Check sheet for the modelled part. Datum: model origin and axes. Units: mm. A direction names the side the tool comes from. Give positions to 0.01 mm unless a question says otherwise; leave off trailing zeros. Loops run counter-clockwise (first coordinate to the right, second up) from the corner with the lowest first, then second, coordinate; pieces in that order, holes last. Notation, with made-up numbers: (30.25, 55.25) - (69.25, 55.25) arc R11 ccw to (69.25, 72.25) - close; hole circle Ø2 at (77, 7). An arc over 180 degrees is marked (long way). Answer in a Markdown table with one row per item. Add a question column.
(1) Sectioned sample at C-C on x = -12. Enter the section's corners in (y, z).
(2) Sectioned sample at A-A on y = 10. Enter the section's corners in (x, z), then the cut area to 3 significant figures.
(3) Thickness scan on L1, parallel to X at y = -52, z = 69; L2, parallel to Y at x = -12, z = -12; L3, parallel to Y at x = -41.5, z = 22.5. Record the ranges inside material, lowest first.
(4) Sectioned sample at D-D on z = -18. Enter the section's corners in (x, y), then the cut area to 3 significant figures.
(5) Sectioned sample at B-B on z = 73. Enter the section's corners in (x, y).
(6) Set-up check for faces 4 (the face through (-38, 66.514, 29)), 5 (the face through (-13, -13, -8.321)), 6 (the face through (0, 16, 18)): record each of +Z, -Z, +X, -X, +Y, -Y from which the full face is reachable in a straight line by a thin tool's end or side.
(7) Go/stop test with flat-tipped pins: P1, Ø12.5, axis at x = 15, z = 24.5, coming from the -Y side; P2, Ø2, axis at x = 3, y = -27, coming from the +Z side; P3, Ø12.5, axis at x = -7, z = -55.5, coming from the +Y side. Record where each tip stops, or that it passes through.
(8) Draft check along Z on faces 1 (the face through (-25.4, -7, 46)), 2 (the face through (0, -13, -14)), 3 (the face through (-38, -9, 102.951)). Enter one of: released by +Z, released by -Z, zero draft, split by the parting line, or undercut.
from build123d import *

# Parameters (mm, degrees)
F0_W     = 75.5894184113
F0_H     = 75.1656368375
F0_W_2   = 75.6931006908
F1_DEPTH = 25.4
F2_W     = 58.5926715285
F2_H     = 41.5871664882
F2_W_2   = 8.5760951042
F2_H_2   = 8.3214826882
F2_W_3   = 8.4206517786
F3_DEPTH = 25.4
F4_W     = 91.1564920098
F4_H     = 141.0772651434
F4_H_2   = 8.5697695613
F5_DEPTH = 25.4


with BuildPart() as f1:
    # F0 (on Right) → F1 (new body)
    with BuildSketch(Plane.YZ):
        with Locations((-37.7947092056, 37.5828184187)):
            Rectangle(F0_W, F0_H)
        with Locations((37.8465503454, 37.5828184187)):
            Rectangle(F0_W_2, F0_H)
        Polygon((0, 0), (-75.5894184113, 0), (-75.5894184113, -74.7117847204), (75.6931006908, -74.7117847204), (75.6931006908, 0), align=None)
    extrude(amount=F1_DEPTH)

    # F2 (on face) → F3 (join)
    with BuildSketch(Plane(origin=(0, 0, 0), x_dir=(0, -1, 0), z_dir=(-1, 0, 0))):
        with Locations((46.293082647, -53.9182014763)):
            Rectangle(F2_W, F2_H)
        Polygon((0, -74.7117847204), (16.9967468828, -74.7117847204), (16.9967468828, -33.1246182323), (16.9967468828, -22.4458947778), (0, -22.4458947778), align=None)
        Polygon((16.9967468828, -33.1246182323), (75.5894184113, -33.1246182323), (75.5894184113, -20.1201699674), (16.9967468828, -20.1201699674), (16.9967468828, -22.4458947778), align=None)
        Polygon((16.9967468828, -20.1201699674), (75.5894184113, -20.1201699674), (75.5894184113, 0), (16.9967468828, 0), (16.9967468828, -8.3214826882), align=None)
        Polygon((0, -22.4458947778), (16.9967468828, -22.4458947778), (16.9967468828, -20.1201699674), (8.5760951042, -20.1201699674), (8.5760951042, -8.3214826882), (0, -8.3214826882), align=None)
        with Locations((4.2880475521, -4.1607413441)):
            Rectangle(F2_W_2, F2_H_2)
        with Locations((12.7864209935, -4.1607413441)):
            Rectangle(F2_W_3, F2_H_2)
    extrude(amount=F3_DEPTH)

    # F4 (on face) → F5 (join)
    with BuildSketch(Plane(origin=(-25.4, 0, 0), x_dir=(0, -1, 0), z_dir=(-1, 0, 0))):
        with Locations((-20.9354860708, 23.8422006369)):
            Rectangle(F4_W, F4_H)
        Polygon((24.6427599341, 102.9506027699), (24.6427599341, 94.3808332086), (24.6427599341, -46.6964319348), (82.840628922, -46.6964319348), (82.840628922, 102.9506027699), align=None)
        with Locations((-20.9354860708, 98.6657179892)):
            Rectangle(F4_W, F4_H_2)
    extrude(amount=F5_DEPTH)


solid = f1.part
Reply:
| question | item | result |
|---|---|---|
| 1 | outline | (-75.59, -74.71) - (0, -74.71) - (0, 0) - (-75.59, 0) - close; hole (-17, -20.12) - (-8.58, -20.12) - (-8.58, -8.32) - (-17, -8.32) - close |
| 2 | outline | (-50.8, -46.7) - (-25.4, -46.7) - (-25.4, 102.95) - (-50.8, 102.95) - close; (0, -74.71) - (25.4, -74.71) - (25.4, 75.17) - (0, 75.17) - close |
| 2 | area | 7,610 mm^2 |
| 3 | L1 | -50.8 to -25.4, 0 to 25.4 |
| 3 | L2 | -75.59 to -17, -8.58 to 0 |
| 3 | L3 | -82.84 to 66.51 |
| 4 | outline | (-50.8, -82.84) - (-25.4, -82.84) - (-25.4, -75.59) - (25.4, -75.59) - (25.4, 75.69) - (0, 75.69) - (0, 0) - (-25.4, 0) - (-25.4, 66.51) - (-50.8, 66.51) - close; hole (-25.4, -17) - (0, -17) - (0, -8.58) - (-25.4, -8.58) - close |
| 4 | area | 9,340 mm^2 |
| 5 | outline | (-50.8, -82.84) - (-25.4, -82.84) - (-25.4, 66.51) - (-50.8, 66.51) - close; (0, -75.59) - (25.4, -75.59) - (25.4, 75.69) - (0, 75.69) - close |
| 6 | face 4 | +Z, -Z, -X, +Y |
| 6 | face 5 | none |
| 6 | face 6 | +Z, +Y |
| 7 | P1 | y = -75.59 |
| 7 | P2 | z = 75.17 |
| 7 | P3 | y = 0 |
| 8 | face 1 | zero draft |
| 8 | face 2 | undercut |
| 8 | face 3 | released by +Z |
